Print and shaded views of the part. All mm, measured from the part's lowest x, y and z. A direction names the side the tool comes from. Round coordinates to 2 decimals unless told otherwise and drop trailing zeros. Write each loop counter-clockwise with the first axis right and the second up, starting at its lowest first coordinate (ties: lowest second). Pieces come first, ordered by that corner, then holes. Notation, with made-up numbers: (-25.75, 54.25) - (21.25, 54.25) arc R12 cw to (21.25, 69.25) - close; hole circle Ø9 at (48, 47.5). An arc over 180 degrees is marked (long way). One line per item, written item: value.
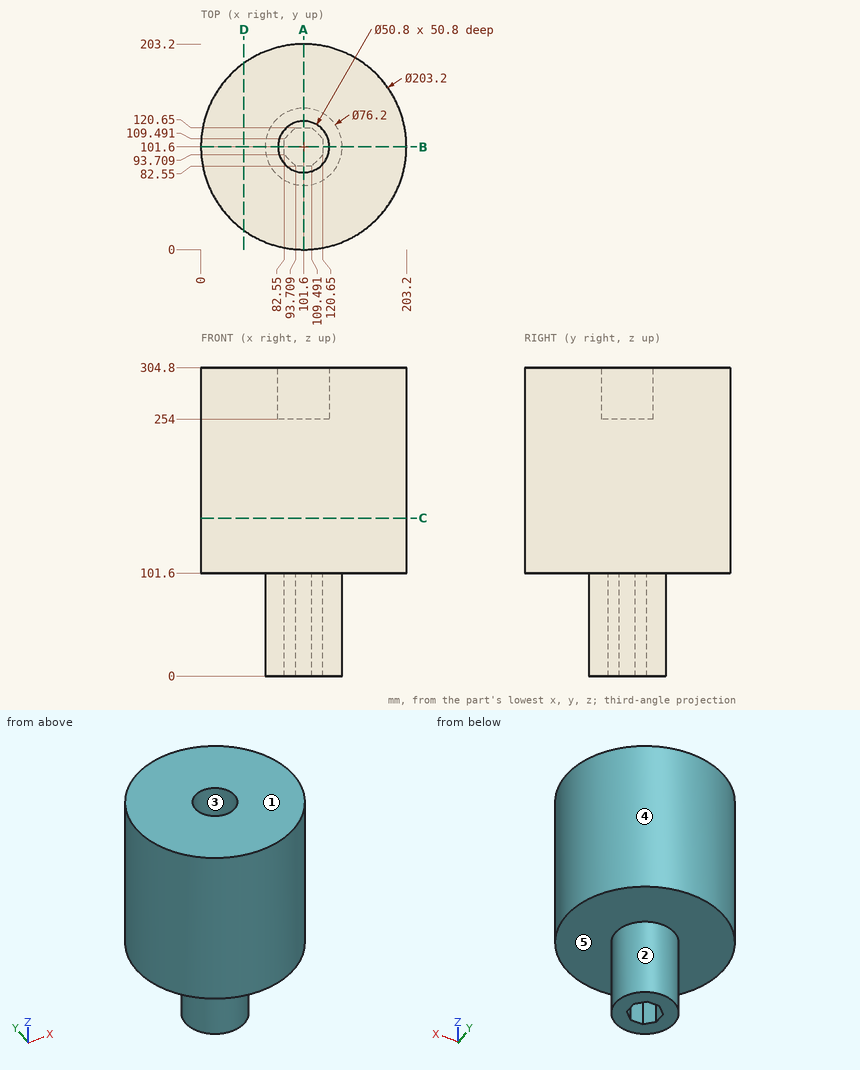
1. Tool access for the marked faces 1 and 2: list every direction of +Z, -Z, +X, -X, +Y, -Y with a clear straight run to the whole face (end or side of a thin tool).
Report:
face 1: +Z, +X, -X, +Y, -Y
face 2: -Z
2. Mould opens along Y. For the marked faces 3, 4 and 5 say: released by +Y, released by -Y, zero draft, split by the parting line, or undercut.
Report:
face 3: undercut
face 4: split by the parting line
face 5: zero draft
3. Wall check: probe 1 along Y at (x, z) = (101.6, 285.5); probe 2 along Z at (x, y) = (167, 92); probe 3 along Y at (x, z) = (83, 260.5). Give the ranges that are in metal, low to high. Write a range as [from, to].
Report:
probe 1: [0, 76.2], [127, 203.2]
probe 2: [101.6, 304.8]
probe 3: [1.72, 84.3], [118.9, 201.48]
4. Band-saw the part on C-C on z = 156. Write the cut outline in (x, y), plus the area to 3 significant figures.
Report:
outline: circle Ø203.2 at (101.6, 101.6)
area: 32,400 mm²
5. Drop flat-ended pins along their axis: pin 1 (17.5 mm diameter, centred on x = 98, z = 73, fed in from -Y); pin 2 (1.5 mm diameter, centred on y = 84, z = 223, fed in from -X); pin 3 (5 mm diameter, centred on x = 78, z = 84, fed in from -Y); pin 4 (5 mm diameter, centred on y = 144, z = 45, fed in from -X) (3 decimals). Give the stop position or say it passes through.
Report:
pin 1: y = 63.5
pin 2: x = 1.41
pin 3: y = 69.88
pin 4: through
6. Band-saw the part on D-D on x = 42.5. Write the cut outline in (y, z), plus the area to 3 significant figures.
Report:
outline: (18.96, 101.6) - (184.24, 101.6) - (184.24, 304.8) - (18.96, 304.8) - close
area: 33,600 mm²
7. Band-saw the part on A-A on x = 101.6. Write the cut outline in (y, z).
Report:
outline: (0, 101.6) - (63.5, 101.6) - (63.5, 0) - (82.55, 0) - (82.55, 101.6) - (120.65, 101.6) - (120.65, 0) - (139.7, 0) - (139.7, 101.6) - (203.2, 101.6) - (203.2, 304.8) - (127, 304.8) - (127, 254) - (76.2, 254) - (76.2, 304.8) - (0, 304.8) - close
